```python
from build123d import *

# Parameters (mm, degrees)
SKETCH1_R           = 31.75
BOSS_EXTRUDE1_DEPTH = 152.4
BOSS_EXTRUDE2_DEPTH = 101.6
FILLET1_R           = 25.4


with BuildPart() as part:
    # Sketch1 → Boss-Extrude1 (new body)
    with BuildSketch(Plane.XY):
        with Locations((0, 95.25)):
            Circle(SKETCH1_R)
    extrude(amount=BOSS_EXTRUDE1_DEPTH)

    # Sketch2 → Boss-Extrude2 (add)
    with BuildSketch(Plane(origin=(0, 0, 0), x_dir=(-1, 0, 0), z_dir=(0, 0, -1))):
        Polygon((-101.6, 177.8), (-152.4, 127), (-152.4, 50.8), (-101.6, 0), (101.6, 0), (152.4, 50.8), (152.4, 127), (101.6, 177.8), align=None)
    extrude(amount=BOSS_EXTRUDE2_DEPTH)

    # Fillet1
    fillet1_edges = [part.edges().sort_by_distance(p)[0] for p in [
        (-31.75, 95.25, 0),
    ]]
    fillet(fillet1_edges, radius=FILLET1_R)


solid = part.part
```
Geometry check sheet. Reference: the model listing, model coordinates, mm. A direction names the side the tool comes from. Coordinates: 2 decimals unless noted, no trailing zeros. Loops run counter-clockwise (first coordinate to the right, second up) from the corner with the lowest first, then second, coordinate; pieces in that order, holes last. Notation, with made-up numbers: (3, -23) - (8, -23) arc R27 ccw to (8, 7) - close; hole circle Ø5 at (41, 21.5). An arc over 180 degrees is marked (long way). One line per item, written item: value. Start each with the question number.
(1) Material ranges on line 1 (Z direction, x = -54.5, y = 25); line 2 (X direction, y = 95, z = 67.5); line 3 (X direction, y = 40.5, z = -60.5), recorded low to high. Write a range as [from, to].
(2) Cross-section at D-D on y = 165.5. Enter the section's corners in (x, z).
(3) Cross-section at B-B on z = -10. Enter the section's corners in (x, y), plus the area to 3 significant figures.
(4) Cross-section at C-C on y = 95.25. Enter the section's corners in (x, z), plus the area to 3 significant figures.
(5) Mould release check, pull along Y, two halves, no side actions. Record for faces 3 (the flat face through (152.4, 89, -50)), 4 (the flat face through (-126.6, 25, -50.1)), 5 (the flat face through (-1, 177.8, -50)): released by +Y, released by -Y, zero draft, split by the parting line, or undercut.
(6) Depth check by flat-ended pin: P1, Ø6, axis at y = 99, z = 9, coming from the -X side; P2, Ø6, axis at y = 39, z = -68, coming from the +X side. Enter the tip coordinate at first touch or a pass-through.
(7) Tool access check on faces 1 (the cylindrical face through (-4.13, 126.73, 88.01)), 2 (the flat face through (127.4, 25.8, -50.1)). Record the directions out of +Z, -Z, +X, -X, +Y, -Y that give a thin tool (end or side, any length) a straight path to the whole face; none if there is none.
(8) Cross-section at A-A on x = 0. Enter the section's corners in (y, z), plus the area to 3 significant figures.
Results below:
1. line 1: z = [-101.6, 0]
1. line 2: x = [-31.75, 31.75]
1. line 3: x = [-142.1, 142.1]
2. outline: (-113.9, -101.6) - (113.9, -101.6) - (113.9, 0) - (-113.9, 0) - close
3. outline: (-152.4, 50.8) - (-101.6, 0) - (101.6, 0) - (152.4, 50.8) - (152.4, 127) - (101.6, 177.8) - (-101.6, 177.8) - (-152.4, 127) - close
3. area: 49,000 mm2
4. outline: (-152.4, -101.6) - (152.4, -101.6) - (152.4, 0) - (57.15, 0) arc R25.4 cw to (31.75, 25.4) - (31.75, 152.4) - (-31.75, 152.4) - (-31.75, 25.4) arc R25.4 cw to (-57.15, 0) - (-152.4, 0) - close
4. area: 40,900 mm2
5. face 3: zero draft
5. face 4: released by -Y
5. face 5: released by +Y
6. P1: stops at x = -40.59
6. P2: stops at x = 143.6
7. face 1: +Z
7. face 2: +Z, -Z, +X, -Y
8. outline: (0, -101.6) - (177.8, -101.6) - (177.8, 0) - (152.4, 0) arc R25.4 cw to (127, 25.4) - (127, 152.4) - (63.5, 152.4) - (63.5, 25.4) arc R25.4 cw to (38.1, 0) - (0, 0) - close
8. area: 28,000 mm2
